Build history of the part. All positions in model axes, mm. Face numbers are marked on the shaded views. A direction names the side the tool comes from. Give positions to 0.01 mm unless a question says otherwise; leave off trailing zeros. Loops run counter-clockwise (first coordinate to the right, second up) from the corner with the lowest first, then second, coordinate; pieces in that order, holes last. Notation, with made-up numbers: (2.25, -5) - (13.25, -5) arc R9 ccw to (13.25, 6) - close; hole circle Ø5 at (-15, 51.5). An arc over 180 degrees is marked (long way). Return JSON: item names as keys, results as strings. Group by question number.
1) Drill centre lines: probe 1 along X at (y, z) = (-5, 0.5); probe 2 along Y at (x, z) = (-2, -2.5); probe 3 along Y at (x, z) = (12.5, 2). Where is each one in solid material? Low to high. Write a range as from..to.
2) Slice it at C-C (x = 0.5). List the corners of the cut face in (y, z).
3) Slice it at B-B (y = -7). List the corners of the cut face in (x, z), and give its area (3 significant figures).
4) Drop flat-ended pins along their axis: pin 1 (5 mm diameter, centred on y = 9.5, z = -3, fed in from -X); pin 2 (2.5 mm diameter, centred on x = -14, z = 2.5, fed in from +Y); pin 3 (6 mm diameter, centred on y = 15.5, z = -1, fed in from -X). Give the stop position or say it passes through.
5) Slice it at A-A (z = -4.25). List the corners of the cut face in (x, y), and give its area (3 significant figures).
6) Slice it at D-D (x = -5). List the corners of the cut face in (y, z).
7) 3-axis set-ups, long thin cutter, end or side, ignore diameter. For the marked faces 1, 2, 3 and 4: which of +Z, -Z, +X, -X, +Y, -Y reach the whole face in a straight line?
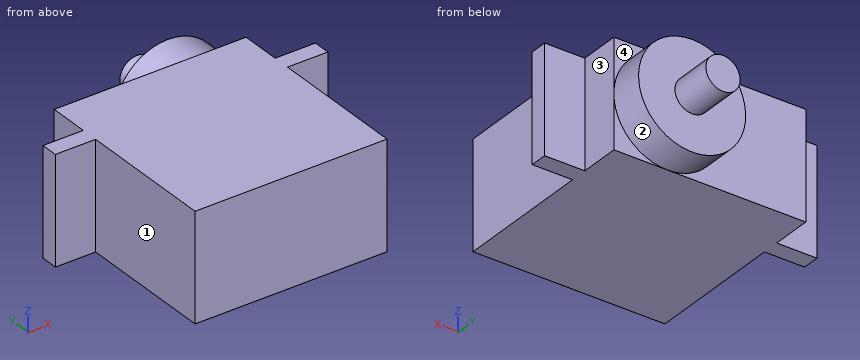
```python
from build123d import *

# Parameters (mm, degrees)
SKETCH_1_W      = 22.4
SKETCH_1_H      = 22.8
EXTRUDE_1_DEPTH = 6.25
SKETCH_4_W      = 4.7
SKETCH_4_H      = 2
EXTRUDE_2_DEPTH = 12.5
SKETCH_5_R      = 6.25
EXTRUDE_3_DEPTH = 4
SKETCH_6_R      = 2
EXTRUDE_4_DEPTH = 5


with BuildPart() as part:
    # 草图1 → 凸台-拉伸1 (new, symmetric)
    with BuildSketch(Plane.XY):
        Rectangle(SKETCH_1_W, SKETCH_1_H)
    extrude(amount=EXTRUDE_1_DEPTH, both=True)

    # 草图4 → 凸台-拉伸2 (add)
    with BuildSketch(Plane.XY.offset(6.25)):
        with Locations((-13.55, 5.7)):
            Rectangle(SKETCH_4_W, SKETCH_4_H)
        with Locations((13.55, 5.7)):
            Rectangle(SKETCH_4_W, SKETCH_4_H)
    extrude(amount=-EXTRUDE_2_DEPTH)

    # 草图5 → 凸台-拉伸3 (add)
    with BuildSketch(Plane(origin=(0, 11.4, 0), x_dir=(1, 0, 0), z_dir=(0, 1, 0))):
        with Locations(Location((4.95, 0, 0), (0, 0, 270))):
            Circle(SKETCH_5_R)
    extrude(amount=EXTRUDE_3_DEPTH)

    # 草图6 → 凸台-拉伸4 (add)
    with BuildSketch(Plane(origin=(0, 15.4, 0), x_dir=(1, 0, 0), z_dir=(0, 1, 0))):
        with Locations(Location((4.95, 0, 0), (0, 0, 270))):
            Circle(SKETCH_6_R)
    extrude(amount=EXTRUDE_4_DEPTH)


solid = part.part
```
Results:
{
 "1": {"probe 1": "-11.2..11.2", "probe 2": "-11.4..11.4", "probe 3": "4.7..6.7"},
 "2": {"outline": "(-11.4, -6.25) - (11.4, -6.25) - (11.4, -4.39) - (15.4, -4.39) - (15.4, 4.39) - (11.4, 4.39) - (11.4, 6.25) - (-11.4, 6.25) - close"},
 "3": {"outline": "(-11.2, -6.25) - (11.2, -6.25) - (11.2, 6.25) - (-11.2, 6.25) - close", "area": "280 mm2"},
 "4": {"pin 1": "x = -11.2", "pin 2": "y = 6.7", "pin 3": "x = -1.3"},
 "5": {"outline": "(-15.9, 4.7) - (-11.2, 4.7) - (-11.2, -11.4) - (11.2, -11.4) - (11.2, 4.7) - (15.9, 4.7) - (15.9, 6.7) - (11.2, 6.7) - (11.2, 11.4) - (9.53, 11.4) - (9.53, 15.4) - (0.37, 15.4) - (0.37, 11.4) - (-11.2, 11.4) - (-11.2, 6.7) - (-15.9, 6.7) - close", "area": "566 mm2"},
 "6": {"outline": "(-11.4, -6.25) - (11.4, -6.25) - (11.4, 6.25) - (-11.4, 6.25) - close"},
 "7": {"face 1": "+Z, -Z, -X, -Y", "face 2": "+Y", "face 3": "+Z, -Z, +X, +Y", "face 4": "+Z, +X, +Y"}
}
